from build123d import *

# Parameters (mm, degrees)
SKETCH_1_W          = 50
SKETCH_1_H          = 40
EXTRUDE_1_DEPTH     = 85
CUT_EXTRUDE_1_DEPTH = 60
EXTRUDE_2_DEPTH     = 25
SKETCH_4_W          = 50
SKETCH_4_H          = 27
EXTRUDE_3_DEPTH     = 5


with BuildPart() as part:
    # 草图1 → 凸台-拉伸1 (new body)
    with BuildSketch(Plane(origin=(0, 0, 0), x_dir=(0, 0, -1), z_dir=(1, 0, 0))):
        with Locations((-25, 20)):
            Rectangle(SKETCH_1_W, SKETCH_1_H)
    extrude(amount=EXTRUDE_1_DEPTH)

    # 草图2 → 切除-拉伸1 (cut)
    with BuildSketch(Plane(origin=(0, 40, 0), x_dir=(1, 0, 0), z_dir=(0, 1, 0))):
        Polygon((45, -7), (0, -7), (0, -35), (0, -43), (80, -43), (80, -33), (45, -33), align=None)
    extrude(amount=-CUT_EXTRUDE_1_DEPTH, mode=Mode.SUBTRACT)

    # 草图3 → 凸台-拉伸2 (add)
    with BuildSketch(Plane.XZ):
        Polygon((0, 43), (45, 43), (80, 43), (80, 33), (45, 33), (45, 28), (0, 28), align=None)
    extrude(amount=-EXTRUDE_2_DEPTH)

    # 草图4 → 凸台-拉伸3 (add)
    with BuildSketch(Plane.ZY):
        with Locations((25, 13.5)):
            Rectangle(SKETCH_4_W, SKETCH_4_H)
    extrude(amount=EXTRUDE_3_DEPTH)


solid = part.part
Source: CAD feature listing. Evaluate the final solid. Frame: model axes, mm. A direction names the side the tool comes from. Round coordinates to 2 decimals unless told otherwise and drop trailing zeros. Loops run counter-clockwise (first coordinate to the right, second up) from the corner with the lowest first, then second, coordinate; pieces in that order, holes last. Notation, with made-up numbers: (80, -18) - (96, -18) arc R27 ccw to (96, 14) - close; hole circle Ø7 at (-38.5, -4). An arc over 180 degrees is marked (long way). Write item = value, one per line. Start each with the question number.
(1) Section query D-D, the plane x = 75.5. Output: boundary loops of the cut face in (y, z), plus the area to 3 significant figures.
(2) Pull-direction query (X, two-part tool) for faces 4 (the face through (45, 20, 17)), 5 (the face through (51, 40, 20)), 6 (the face through (0, 34, 4)), 7 (the face through (41, 25, 37)); classes: +X half, -X half, draft (parallel to the pull), parting line (faces both ways), or undercut.
(3) Set-up query: faces 1 (the face through (51, 0, 25)), 2 (the face through (0, 33, 46)), 3 (the face through (23, 20, 7)). Return all of +Z, -Z, +X, -X, +Y, -Y with unobstructed straight access to the full face (end or side cutting, diameter ignored); none if empty.
(4) Section query C-C, the plane z = 10. Output: boundary loops of the cut face in (x, y), plus the area to 4 significant figures.
(5) Section query A-A, the plane x = 41. Output: boundary loops of the cut face in (y, z).
(6) Ray query, line 1 along Z through (x, y) = (12.5, 11); line 2 along X through (y, z) = (12, 10); line 3 along Z through (x, y) = (48, 37.5). Return the intervals inside material, ascending. Write a range as from..to.
(7) Section query B-B, the plane y = 8.5. Output: boundary loops of the cut face in (x, z), plus the area to 4 significant figures.
(8) Pin query (flat end, axial travel): pin 1 (2.5 mm diameter, centred on x = -2, z = 25, fed in from +Y); pin 2 (2 mm diameter, centred on y = 33, z = 4.5, fed in from -X); pin 3 (2 mm diameter, centred on x = 13, z = 31.5, fed in from +Y). Return the tip coordinate at first contact, or that it passes through.
Conclusion:
q1.outline = (0, 0) - (40, 0) - (40, 33) - (25, 33) - (25, 43) - (40, 43) - (40, 50) - (0, 50) - close
q1.area = 1,850 mm2
q2.face_4 = undercut
q2.face_5 = draft
q2.face_6 = -X half
q2.face_7 = undercut
q3.face_1 = +Z, -Z, +X, -X, -Y
q3.face_2 = +Z, -Z, -X, +Y
q3.face_3 = +Y, -Y
q4.outline = (-5, 0) - (0, 0) - (0, 27) - (-5, 27) - close; (45, 0) - (85, 0) - (85, 40) - (45, 40) - close
q4.area = 1,735 mm2
q5.outline = (0, 0) - (40, 0) - (40, 7) - (0, 7) - close; (0, 28) - (25, 28) - (25, 43) - (40, 43) - (40, 50) - (0, 50) - close
q6.line_1 = 0..7, 28..50
q6.line_2 = -5..0, 45..85
q6.line_3 = 0..33, 43..50
q7.outline = (-5, 0) - (85, 0) - (85, 50) - (-5, 50) - close; hole (0, 7) - (45, 7) - (45, 28) - (0, 28) - close
q7.area = 3,555 mm2
q8.pin_1 = 27
q8.pin_2 = 0
q8.pin_3 = 25
